```python
from build123d import *

# Parameters (mm, degrees)
F0_R           = 25
F0_R_2         = 10.5
F1_DEPTH       = 4
F2_R           = 10.5
F3_DEPTH       = 10
F5_D           = 4
F5_CSINK_D     = 7
F5_CSINK_ANGLE = 90
F7_D           = 4


with BuildPart() as f1:
    # F0 (on Top) → F1 (new body)
    with BuildSketch(Plane.XY):
        Circle(F0_R)
        Circle(F0_R_2, mode=Mode.SUBTRACT)
    extrude(amount=F1_DEPTH)

    # F2 (on face) → F3 (join)
    with BuildSketch(Plane.XY.offset(4)):
        with BuildLine():
            Line((-5, -12), (5, -12))
            ThreePointArc((5, -12), (13, 0), (5, 12))
            Line((5, 12), (-5, 12))
            ThreePointArc((-5, 12), (-13, 0), (-5, -12))
        make_face()
        Circle(F2_R, mode=Mode.SUBTRACT)
    extrude(amount=F3_DEPTH)

    # F5 (through all)
    with Locations(Plane.XY.offset(4)):
        with Locations((-10, -17.320508), (-10, 17.320508), (20, 0)):
            CounterSinkHole(F5_D / 2, F5_CSINK_D / 2, counter_sink_angle=F5_CSINK_ANGLE)

    # F7 (through all)
    with Locations(Plane.XZ.offset(12)):
        with Locations((0, 9)):
            Hole(F7_D / 2)


solid = f1.part
```
Design review of the part built by this model. Coordinates are the model's own, in mm. A direction names the side the tool comes from. Coordinates: 2 decimals unless noted, no trailing zeros. Loops run counter-clockwise (first coordinate to the right, second up) from the corner with the lowest first, then second, coordinate; pieces in that order, holes last. Notation, with made-up numbers: M 42,7.25 L 96,7.25 A23 ccw 96,35.25 Z; hole C 65.5,27 d10. An arc over 180 degrees is marked long. One line per question, with ' | ' between items.
(1) We need section C-C (y = 6). Give the boundary of the cut face in (x, z).
Filled in:
outline: M -24.27,0 L -8.62,0 L -8.62,14 L -11.53,14 L -11.53,4 L -24.27,4 Z; M 8.62,0 L 24.27,0 L 24.27,4 L 11.53,4 L 11.53,14 L 8.62,14 Z
(2) For pin 1 Ø5 at (x, z) = (0, 9) entering from -Y; pin 2 Ø3 at (x, z) = (0, 9) entering from +Y; pin 3 Ø1.5 at (y, z) = (7, 3.5) entering from +X; pin 4 Ø4 at (x, z) = (-0.5, 3) entering from -Y, all flat-tipped, find the tip position at first contact; note any pin that passes through.
Filled in:
pin 1: stops at y = -12 | pin 2: passes through | pin 3: stops at x = 24.21 | pin 4: stops at y = -25
(3) We need section A-A (z = 9). Give the boundary of the cut face in (x, y), and give its area (3 significant figures).
Filled in:
outline: M -5,-12 L -2,-12 L -2,-10.31 A10.5 cw -2,10.31 L -2,12 L -5,12 A13 ccw Z; M 2,-12 L 5,-12 A13 ccw 5,12 L 2,12 L 2,10.31 A10.5 cw 2,-10.31 Z | area: 159 mm^2
(4) Machinability: for faces 4 (the face through (-2.2, 12, 8.9)), 5 (the face through (2.2, -12, 8.9)), 6 (the face through (13, 0, 9)), which of the approach directions +Z, -Z, +X, -X, +Y, -Y give a long, thin tool a straight path to every point of the face, cutting with its end or side? Answer none if there is none.
Filled in:
face 4: +Z, +X, -X, +Y | face 5: +Z, +X, -X, -Y | face 6: +Z, +X
(5) We need section D-D (z = 12.5). Give the boundary of the cut face in (x, y), and give its area (3 significant figures).
Filled in:
outline: M -5,-12 L 5,-12 A13 ccw 5,12 L -5,12 A13 ccw Z; hole C 0,0 d21 | area: 171 mm^2
(6) Wall thickness on probe 1 along Z at (x, y) = (0, -11.4); probe 2 along Z at (x, y) = (-11, 10.5); probe 3 along Y at (x, z) = (7, 2.75): over which ranges is each line inside the solid? List them lowest first.
Filled in:
probe 1: z = 0 to 7, 11 to 14 | probe 2: z = 0 to 4 | probe 3: y = -24 to -7.83, 7.83 to 24
(7) Draft analysis for pull direction X (two halves, no side actions). For faces 1 (the face through (11, -11, 4)), 2 (the face through (21.6, -1.2, 1.2)), 3 (the face through (-13, 0, 9)), state which applies: released by +X, released by -X, zero draft, split by the parting line, or undercut.
Filled in:
face 1: zero draft | face 2: undercut | face 3: released by -X
(8) We need section B-B (x = 20). Give the boundary of the cut face in (y, z).
Filled in:
outline: M -15,0 L -2,0 L -2,2.5 L -3.5,4 L -15,4 Z; M 2,0 L 15,0 L 15,4 L 3.5,4 L 2,2.5 Z
